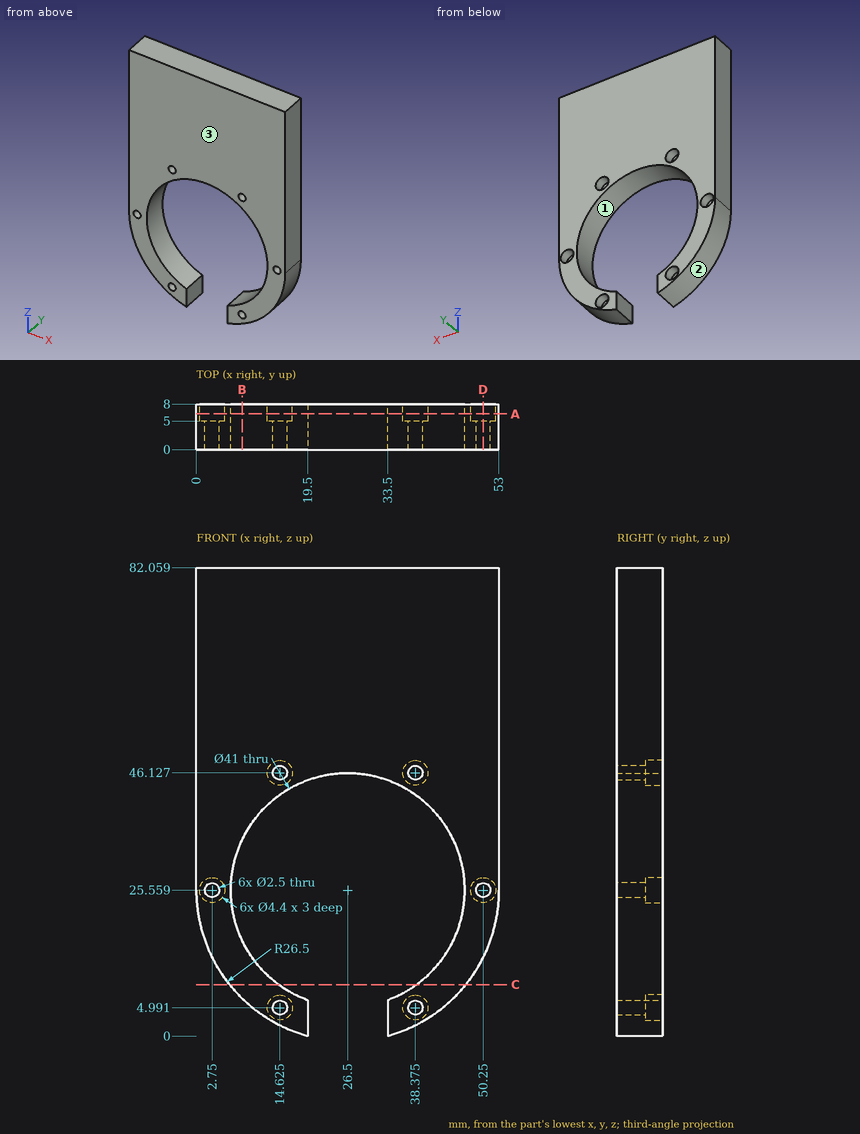
Source: three-view drawing plus pictorial views. Frame: mm from the lowest corner of the part. Round coordinates to 2 decimals unless told otherwise and drop trailing zeros. Loops run counter-clockwise (first coordinate to the right, second up) from the corner with the lowest first, then second, coordinate; pieces in that order, holes last. Notation, with made-up numbers: M 3.5,-19 L 19.5,-19 A19 ccw 19.5,13 Z; hole C 55,47.5 d7. An arc over 180 degrees is marked long. Put each result on its own line as item: value. Start each with the question number.
(1) Section query C-C (z = 9). Return loops of the section in (x, y) (1 decimal), then the cut area to 3 significant figures.
(2) Section query A-A (y = 6.25). State how many separate pieces and enclosed holes the cut face has, then the cut area to 3 significant figures.
(3) Contact query for flat-ended pins moving along their axis: pin 1 Ø4 at (x, z) = (50.25, 25.56) entering from -Y; pin 2 Ø3 at (x, z) = (38.38, 4.99) entering from +Y; pin 3 Ø2 at (x, y) = (31.5, 4) entering from -Z; pin 4 Ø2 at (y, z) = (1, 11) entering from -X. Output: stop coordinate, or through.
(4) Section query B-B (x = 8). Return loops of the section in (y, z) (1 decimal).
(5) Draft query along Z for the marked faces 1, 2 and 3. Return one class per face: +Z half, -Z half, draft (parallel to the pull), parting line (faces both ways), or undercut.
(6) Material intervals for line 1 along X through (y, z) = (6, 26) (1 decimal); line 2 along X through (y, z) = (3.5, 24.5) (1 decimal); line 3 along Z through (x, y) = (18, 7.25) (1 decimal), sorted ascending. Write a range as [from, to].
(7) Section query D-D (x = 50.25). Return loops of the section in (y, z).
Findings below:
1. outline: M 5.8,0 L 14.4,0 L 14.4,8 L 5.8,8 Z; M 38.6,0 L 47.2,0 L 47.2,8 L 38.6,8 Z
1. area: 138 mm2
2. separate pieces: 1
2. enclosed holes: 6
2. area: 2,600 mm2
3. pin 1: stops at y = 0
3. pin 2: stops at y = 5
3. pin 3: stops at z = 45.16
3. pin 4: stops at x = 3.73
4. outline: M 0,6.6 L 8,6.6 L 8,16.7 L 0,16.7 Z; M 0,34.4 L 8,34.4 L 8,82.1 L 0,82.1 Z
5. face 1: undercut
5. face 2: -Z half
5. face 3: draft
6. line 1: x = [0, 0.6], [4.9, 6], [47, 48.1], [52.4, 53]
6. line 2: x = [0, 2.1], [3.4, 6], [47, 49.6], [50.9, 53]
6. line 3: z = [0.5, 6.9], [44.2, 82.1]
7. outline: M 0,13.8 L 8,13.8 L 8,23.36 L 5,23.36 L 5,24.31 L 0,24.31 Z; M 0,26.81 L 5,26.81 L 5,27.76 L 8,27.76 L 8,82.06 L 0,82.06 Z
